The listing builds one solid part. Answer for the finished solid, in the listing's coordinates (mm). Face numbers are marked on the shaded views. A direction names the side the tool comes from. Round coordinates to 2 decimals unless told otherwise and drop trailing zeros. Order: outer loops, then holes, each group sorted by start corner. A loop starts at its lowest first (then second) coordinate and runs counter-clockwise, first axis right, second up. Notation, with made-up numbers: (-20, 86) -> (26, 86) arc R27 ccw to (26, 103) -> close; hole circle Ø2 at (40.25, 54.25). An arc over 180 degrees is marked (long way). Answer in a Markdown table with one row per item. Add a question column.
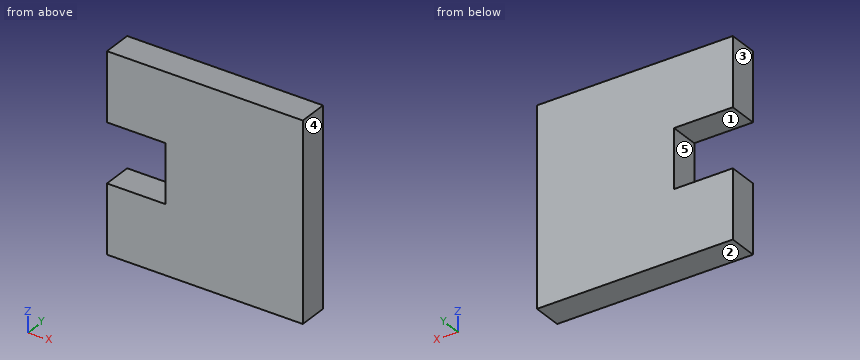
```python
from build123d import *

# Parameters (mm, degrees)
SKIZZE1_W                            = 100
SKIZZE1_H                            = 15
AUFSATZ_LINEAR_AUSTRAGEN1_DEPTH      = 50
SCHNITT_LINEAR_AUSTRAGEN1_DEPTH      = 72.107313267
SCHNITT_LINEAR_AUSTRAGEN1_DEPTH_BACK = 72.107313267
SKIZZE2_W                            = 30
SKIZZE2_H                            = 30


with BuildPart() as part:
    # Skizze1 → Aufsatz-Linear austragen1 (new, symmetric)
    with BuildSketch(Plane.XY):
        Rectangle(SKIZZE1_W, SKIZZE1_H)
    extrude(amount=AUFSATZ_LINEAR_AUSTRAGEN1_DEPTH, both=True)

    # Skizze2 → Schnitt-Linear austragen1 (cut, two sides: drawn at the far end of the back side and taken through both)
    with BuildSketch(Plane(origin=(0, 0, 0), x_dir=(1, 0, 0), z_dir=(0, 1, 0)).offset(-SCHNITT_LINEAR_AUSTRAGEN1_DEPTH_BACK)):
        with Locations((-35, 0)):
            Rectangle(SKIZZE2_W, SKIZZE2_H)
    extrude(amount=SCHNITT_LINEAR_AUSTRAGEN1_DEPTH + SCHNITT_LINEAR_AUSTRAGEN1_DEPTH_BACK, mode=Mode.SUBTRACT)


solid = part.part
```
1. The mould has two halves that part along Z. Classify the marked faces 1, 2 and 3: released by +Z, released by -Z, zero draft, split by the parting line, or undercut.
2. Straight lines are drawn through the part: line 1 along Z through (x, y) = (-39, -5); line 2 along X through (y, z) = (1.75, 7). For each, find the intervals that lie inside material, in ascending order.
3. The part is cut by section B-B (y = -1.25). Give the vertices of the cut face in (x, z).
4. The part is cut by section A-A (x = -30). Give the vertices of the cut face in (y, z).
5. This flat-tipped pin is pushed along its axis until it touches: pin 1 (4.5 mm diameter, centred on y = -1.5, z = 5.5, fed in from -X). Where does it stop, or does it pass through?
6. For the marked faces 4 and 5, determine the directions among +Z, -Z, +X, -X, +Y, -Y from which every point of the face is accessible in a straight line to the end or side of a thin tool.
7. The part is cut by section C-C (z = -9). Give the vertices of the cut face in (x, y), then the cut area to 3 significant figures.
Report:
| question | item | result |
|---|---|---|
| 1 | face 1 | undercut |
| 1 | face 2 | released by -Z |
| 1 | face 3 | zero draft |
| 2 | line 1 | z = -50 to -15, 15 to 50 |
| 2 | line 2 | x = -20 to 50 |
| 3 | outline | (-50, -50) -> (50, -50) -> (50, 50) -> (-50, 50) -> (-50, 15) -> (-20, 15) -> (-20, -15) -> (-50, -15) -> close |
| 4 | outline | (-7.5, -50) -> (7.5, -50) -> (7.5, -15) -> (-7.5, -15) -> close; (-7.5, 15) -> (7.5, 15) -> (7.5, 50) -> (-7.5, 50) -> close |
| 5 | pin 1 | stops at x = -20 |
| 6 | face 4 | +Z, -Z, +X, +Y, -Y |
| 6 | face 5 | -X, +Y, -Y |
| 7 | outline | (-20, -7.5) -> (50, -7.5) -> (50, 7.5) -> (-20, 7.5) -> close |
| 7 | area | 1,050 mm^2 |
